Geometry: final body of the model. Coordinates: model frame, mm. A direction names the side the tool comes from. Coordinates: 2 decimals unless noted, no trailing zeros. Loops run counter-clockwise (first coordinate to the right, second up) from the corner with the lowest first, then second, coordinate; pieces in that order, holes last. Notation, with made-up numbers: (-8, 67.25) - (37, 67.25) arc R26 ccw to (37, 88.25) - close; hole circle Ø9 at (41.25, 30). An arc over 180 degrees is marked (long way). Put each result on its own line as item: value. Start each with the question number.
1) Material intervals for line 1 along Y through (x, z) = (39.5, 1.25); line 2 along X through (y, z) = (42, 1.65); line 3 along X through (y, z) = (26.5, 1.4), sorted ascending. Write a range as from..to.
2) Section B-B on y = 43. Output: boundary loops of the cut face in (x, z), and give its area (3 significant figures).
3) Reachability of faces 1 (the flat face through (82, 0, 1)), 2 (the flat face through (137, -2, 2)), 3 (the flat face through (-2, 70, 2)), 4 (the flat face through (7, -1, 2)), 5 (the flat face through (137, 72, 2)) from +Z, -Z, +X, -X, +Y, -Y: full face, straight path, thin tool, end or side. Return the list, or none.
4) Contact query for flat-ended pins moving along their axis: pin 1 Ø0.9 at (y, z) = (3.5, 2) entering from -X; pin 2 Ø1.5 at (x, z) = (-2, 2) entering from -Y; pin 3 Ø0.9 at (x, z) = (4.5, 1) entering from -Y. Output: stop coordinate, or through.
5) Draft query along X for faces 6 (the flat face through (140, 35.5, 2)), 7 (the flat face through (144, 23, 1)), 8 (the flat face through (4, 26, 2)). Return one class per face: +X half, -X half, draft (parallel to the pull), parting line (faces both ways), or undercut.
6) Section A-A on z = 2.55. Count the separate pieces of the cut face and the enclosed holes in it, and give its area (3 significant figures).
7) Section C-C on x = 105. Output: boundary loops of the cut face in (y, z), and give its area (3 significant figures).
Autodesk Inventor part; units mm, degrees
ref_plane "YZ Plane" through (0, 0, 0) normal (1, 0, 0) x (0, 1, 0)
ref_plane "XZ Plane" through (0, 0, 0) normal (0, 1, 0) x (-1, 0, 0)
ref_plane "XY Plane" through (0, 0, 0) normal (0, 0, 1) x (1, 0, 0)
sketch "Sketch1" plane through (0, 0, 0) normal (0, 0, 1) x (1, 0, 0)
  line L0 (0, 0) -> (144, 0)
  line L1 (144, 0) -> (144, 77)
  line L2 (144, 77) -> (0, 77)
  line L3 (0, 77) -> (0, 0)
  dimension "d0" = 144
  dimension "d1" = 77
extrude "Extrusion1" add sketch "Sketch1" along normal blind 3
sketch "Sketch2" plane through (0, 0, 3) normal (0, 0, 1) x (1, 0, 0)
  line L0 (144, 77) -> (0, 77)
  line L1 (0, 0) -> (144, 0)
  line L2 (0, 77) -> (144, 77)
  line L3 (144, 77) -> (144, 0)
  line L4 (144, 0) -> (0, 0)
  line L5 (0, 0) -> (0, 77)
  line L6 (7, 0) -> (7, -3)
  line L7 (7, -3) -> (17, -3)
  line L8 (17, -3) -> (17, 0)
  line L9 (27, 0) -> (27, -3)
  line L10 (27, -3) -> (37, -3)
  line L11 (37, -3) -> (37, 0)
  line L12 (47, 0) -> (47, -3)
  line L13 (47, -3) -> (57, -3)
  line L14 (57, -3) -> (57, 0)
  line L15 (67, 0) -> (67, -3)
  line L16 (67, -3) -> (77, -3)
  line L17 (77, -3) -> (77, 0)
  line L18 (87, 0) -> (87, -3)
  line L19 (87, -3) -> (97, -3)
  line L20 (97, -3) -> (97, 0)
  line L21 (107, 0) -> (107, -3)
  line L22 (107, -3) -> (117, -3)
  line L23 (117, -3) -> (117, 0)
  line L24 (127, 0) -> (127, -3)
  line L25 (127, -3) -> (137, -3)
  line L26 (137, -3) -> (137, 0)
  line L27 (0, 77) -> (0, 0)
  line L28 (0, 10) -> (-3, 10)
  line L29 (-3, 10) -> (-3, 20)
  line L30 (-3, 20) -> (0, 20)
  line L31 (-3, 40) -> (0, 40)
  line L32 (-3, 30) -> (-3, 40)
  line L33 (0, 30) -> (-3, 30)
  line L34 (-3, 60) -> (0, 60)
  line L35 (-3, 50) -> (-3, 60)
  line L36 (0, 50) -> (-3, 50)
  line L37 (144, 77) -> (0, 77)
  line L38 (0, 77) -> (-3, 77)
  line L39 (-3, 77) -> (-3, 70)
  line L40 (-3, 70) -> (0, 70)
  line L41 (144, 0) -> (144, 77)
  line L42 (144, 77) -> (147, 77)
  line L43 (147, 77) -> (147, 70)
  line L44 (147, 70) -> (144, 70)
  line L45 (144, 0) -> (144, 77)
  line L46 (144, 60) -> (147, 60)
  line L47 (147, 60) -> (147, 50)
  line L48 (147, 50) -> (144, 50)
  line L49 (144, 40) -> (147, 40)
  line L50 (147, 40) -> (147, 30)
  line L51 (147, 30) -> (144, 30)
  line L52 (144, 20) -> (147, 20)
  line L53 (147, 20) -> (147, 10)
  line L54 (147, 10) -> (144, 10)
  dimension "d4" = 3
  dimension "d5" = 10
  dimension "d8" = 20
  dimension "d13" = 3
  dimension "d14" = 10
  dimension "d17" = 20
  dimension "d22" = 3
  dimension "d23" = 7
  dimension "d24" = 3
extrude "Extrusion2" add sketch "Sketch2" against normal blind 3 contours L42 L43 L44 L3 | L5 L40 L39 L38 | L46 L47 L48 L3 | L5 L36 L35 L34 | L49 L50 L51 L3 | L5 L33 L32 L31 | L52 L53 L54 L3 | L5 L28 L29 L30 | L26 L25 L24 L1 | L1 L8 L7 L6 | L23 L22 L21 L1 | L1 L11 L10 L9 | L20 L19 L18 L1 | L1 L14 L13 L12 | L17 L16 L15 L1
sketch "Sketch3" plane through (0, 0, 3) normal (0, 0, 1) x (1, 0, 0)
  line L0 (0, 73.5) -> (7, 73.5)
  line L1 (7, 73.5) -> (7, 70.5)
  line L2 (7, 70.5) -> (0, 70.5)
  line L3 (0, 70.5) -> (0, 73.5)
  line L4 (137, 73.5) -> (144, 73.5)
  line L5 (144, 73.5) -> (144, 70.5)
  line L6 (144, 70.5) -> (137, 70.5)
  line L7 (137, 70.5) -> (137, 73.5)
  line L8 (0, 35.5) -> (7, 35.5)
  line L9 (7, 35.5) -> (7, 32.5)
  line L10 (7, 32.5) -> (0, 32.5)
  line L11 (0, 32.5) -> (0, 35.5)
  line L12 (137, 35.5) -> (144, 35.5)
  line L13 (144, 35.5) -> (144, 32.5)
  line L14 (144, 32.5) -> (137, 32.5)
  line L15 (137, 32.5) -> (137, 35.5)
  line L16 (7, 29) -> (7, 26)
  line L17 (7, 26) -> (0, 26)
  line L18 (0, 26) -> (0, 29)
  line L19 (0, 29) -> (7, 29)
  line L20 (144, 35.5) -> (144, 32.5)
  line L21 (144, 32.5) -> (137, 32.5)
  line L22 (137, 32.5) -> (137, 35.5)
  line L23 (137, 35.5) -> (144, 35.5)
  line L24 (144, 29) -> (144, 26)
  line L25 (144, 26) -> (137, 26)
  line L26 (137, 26) -> (137, 29)
  line L27 (137, 29) -> (144, 29)
  line L28 (-3, 77) -> (147, 77)
  point P0 (0, 0)
  dimension "d27" = 7
  dimension "d28" = 3
  dimension "d31" = 137
  dimension "d34" = 38
  dimension "d41" = 6.5
  dimension "d44" = 137
  dimension "d47" = 3.5
  dimension "d48" = 3.5
extrude "Extrusion3" cut sketch "Sketch3" against normal through all
properties part number "DoosjeVoorkant" material "Wood (Cherry)"
Answer block:
1. line 1: y = 0..77
1. line 2: x = 0..144
1. line 3: x = 7..137
2. outline: (0, 0) - (144, 0) - (144, 3) - (0, 3) - close
2. area: 432 mm²
3. face 1: +Z, -Z, -Y
3. face 2: +Z, -Z, +X, -Y
3. face 3: +Z, -Z, -X
3. face 4: +Z, -Z, -X, -Y
3. face 5: +Z, -Z
4. pin 1: stops at x = 0
4. pin 2: stops at y = 10
4. pin 3: stops at y = 0
5. face 6: undercut
5. face 7: +X half
5. face 8: draft
6. separate pieces: 1
6. enclosed holes: 4
6. area: 11,400 mm²
7. outline: (0, 0) - (77, 0) - (77, 3) - (0, 3) - close
7. area: 231 mm²
